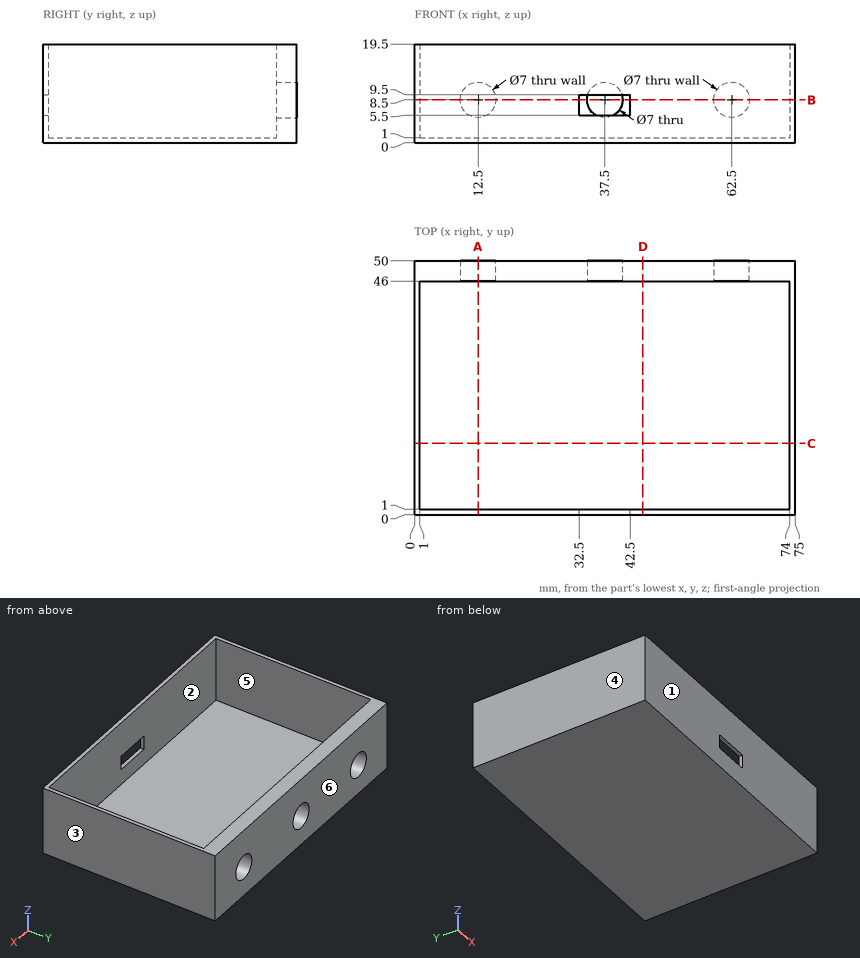
Geometry: see drawing. Coordinates: mm, zero at the bounding-box minimum. A direction names the side the tool comes from. Round coordinates to 2 decimals unless told otherwise and drop trailing zeros. Loops run counter-clockwise (first coordinate to the right, second up) from the corner with the lowest first, then second, coordinate; pieces in that order, holes last. Notation, with made-up numbers: (60, 9.5) -> (89, 9.5) arc R10 ccw to (89, 24.5) -> close; hole circle Ø1 at (5, -33.75). An arc over 180 degrees is marked (long way). Use one line per item in the form item = value. Start each with the question number.
Item 1: Mould query, pull axis X, two halves, no side actions, for the marked faces 1, 2, 3 and 4. Classes: pulls with the +X half, pulls with the -X half, needs draft (parallel to the pull), parting line crosses it, or undercut.
Item 2: Section query C-C on y = 14. Return the cut outline in (x, z).
Item 3: Section query B-B on z = 8.5. Return the cut outline in (x, y), then the cut area to 3 significant figures.
Item 4: Section query D-D on x = 45. Return the cut outline in (y, z), then the cut area to 4 significant figures.
Item 5: Contact query for a flat-ended pin moving along its axis: pin 1 Ø4 at (x, z) = (37.5, 8.5) entering from +Y. Output: stop coordinate, or through.
Item 6: Set-up query: the marked faces 5 and 6. Return all of +Z, -Z, +X, -X, +Y, -Y with unobstructed straight access to the full face (end or side cutting, diameter ignored); none if empty.
Item 7: Material intervals for L1, parallel to Y at x = 51.5, z = 4.25; L2, parallel to X at y = 11, z = 10.5; L3, parallel to Z at x = 62.5, y = 49.15, sorted ascending. Write a range as from..to.
Item 8: Section query A-A on x = 12.5. Return the cut outline in (y, z).
Ans:
q1.face_1 = needs draft
q1.face_2 = undercut
q1.face_3 = pulls with the +X half
q1.face_4 = pulls with the -X half
q2.outline = (0, 0) -> (75, 0) -> (75, 19.5) -> (74, 19.5) -> (74, 1) -> (1, 1) -> (1, 19.5) -> (0, 19.5) -> close
q3.outline = (0, 0) -> (32.5, 0) -> (32.5, 1) -> (1, 1) -> (1, 46) -> (9, 46) -> (9, 50) -> (0, 50) -> close; (16, 46) -> (34, 46) -> (34, 50) -> (16, 50) -> close; (41, 46) -> (59, 46) -> (59, 50) -> (41, 50) -> close; (42.5, 0) -> (75, 0) -> (75, 50) -> (66, 50) -> (66, 46) -> (74, 46) -> (74, 1) -> (42.5, 1) -> close
q3.area = 371 mm^2
q4.outline = (0, 0) -> (50, 0) -> (50, 19.5) -> (46, 19.5) -> (46, 1) -> (1, 1) -> (1, 19.5) -> (0, 19.5) -> close
q4.area = 142.5 mm^2
q5.pin_1 = 1
q6.face_5 = +Z
q6.face_6 = +Z, -Z, +X, -X, +Y
q7.L1 = 0..1, 46..50
q7.L2 = 0..1, 74..75
q7.L3 = 0..5, 12..19.5
q8.outline = (0, 0) -> (50, 0) -> (50, 5) -> (46, 5) -> (46, 1) -> (1, 1) -> (1, 19.5) -> (0, 19.5) -> close; (46, 12) -> (50, 12) -> (50, 19.5) -> (46, 19.5) -> close
